Build history of the part. All positions in model axes, mm. A direction names the side the tool comes from. Round coordinates to 2 decimals unless told otherwise and drop trailing zeros. Loops run counter-clockwise (first coordinate to the right, second up) from the corner with the lowest first, then second, coordinate; pieces in that order, holes last. Notation, with made-up numbers: (54, 55.25) -> (63, 55.25) arc R25 cw to (63, 74.25) -> close; hole circle Ø11 at (12.5, 43). An arc over 180 degrees is marked (long way). Put each result on its own line as item: value. Start each with the question number.
Item 1: Cut at D-D, the plane y = -7. List the corners of the cut face in (x, z), plus the area to 3 significant figures.
Item 2: Drill centre lines: probe 1 along X at (y, z) = (-6, -3.5); probe 2 along X at (y, z) = (-11.5, -10.5); probe 3 along Y at (x, z) = (13, 7). Where is each one in solid material? Low to high. Write a range as [from, to].
Item 3: Cut at B-B, the plane z = -8. List the corners of the cut face in (x, y).
Item 4: Flat gauge pins, fed straight in: pin 1 Ø10 at (x, z) = (32, -7) entering from +Y; pin 2 Ø8 at (x, z) = (14, 4) entering from +Y; pin 3 Ø6 at (x, y) = (22.5, 5) entering from +Z. Where does each tip first touch, or does it go through?
Item 5: Cut at C-C, the plane x = -14.5. List the corners of the cut face in (y, z).
Item 6: Tool access for faces 1 (the cylindrical face through (-19.712, 0.165, -3.746)), 2 (the flat face through (40, -9.4, 0)), 3 (the flat face through (30, -8, 3)): list every direction of +Z, -Z, +X, -X, +Y, -Y with a clear straight run to the whole face (end or side of a thin tool).
Item 7: Cut at A-A, the plane y = 0. List the corners of the cut face in (x, z).
```python
from build123d import *

# Parameters (mm, degrees)
SKETCH1_R           = 18.5
BOSS_EXTRUDE1_DEPTH = 24
SKETCH2_R           = 16
BOSS_EXTRUDE2_DEPTH = 17
SKETCH4_R           = 6
BOSS_EXTRUDE3_DEPTH = 6
SKETCH5_R           = 3
BOSS_EXTRUDE4_DEPTH = 15
SKETCH6_W           = 6.457083565
SKETCH6_H           = 2.403469994
CUT_EXTRUDE1_DEPTH  = 11
SKETCH7_R           = 3.75
BOSS_EXTRUDE5_DEPTH = 5.5


with BuildPart() as part:
    # Sketch1 → Boss-Extrude1 (new body)
    with BuildSketch(Plane(origin=(0, 0, 0), x_dir=(0, 0, -1), z_dir=(1, 0, 0))):
        Circle(SKETCH1_R)
    extrude(amount=BOSS_EXTRUDE1_DEPTH)

    # Sketch2 → Boss-Extrude2 (add)
    with BuildSketch(Plane.ZY):
        Circle(SKETCH2_R)
    extrude(amount=BOSS_EXTRUDE2_DEPTH)

    # Sketch4 → Boss-Extrude3 (add)
    with BuildSketch(Plane(origin=(24, 0, 0), x_dir=(0, 0, -1), z_dir=(1, 0, 0))):
        with Locations((0, -7)):
            Circle(SKETCH4_R)
    extrude(amount=BOSS_EXTRUDE3_DEPTH)

    # Sketch5 → Boss-Extrude4 (add)
    with BuildSketch(Plane(origin=(30, 0, 0), x_dir=(0, 0, -1), z_dir=(1, 0, 0))):
        with Locations((0, -7)):
            Circle(SKETCH5_R)
    extrude(amount=BOSS_EXTRUDE4_DEPTH)

    # Sketch6 → Cut-Extrude1 (cut)
    with BuildSketch(Plane(origin=(45, 0, 0), x_dir=(0, 0, -1), z_dir=(1, 0, 0))):
        with Locations((-0.362875994, -10.601734997)):
            Rectangle(SKETCH6_W, SKETCH6_H)
    extrude(amount=-CUT_EXTRUDE1_DEPTH, mode=Mode.SUBTRACT)

    # Sketch7 → Boss-Extrude5 (add)
    with BuildSketch(Plane.ZY.offset(17)):
        Circle(SKETCH7_R)
    extrude(amount=BOSS_EXTRUDE5_DEPTH)


solid = part.part
```
Reply:
1. outline: (-17, -14.39) -> (0, -14.39) -> (0, -17.12) -> (24, -17.12) -> (24, -6) -> (30, -6) -> (30, -3) -> (45, -3) -> (45, 3) -> (30, 3) -> (30, 6) -> (24, 6) -> (24, 17.12) -> (0, 17.12) -> (0, 14.39) -> (-17, 14.39) -> close
1. area: 1,470 mm^2
2. probe 1: x = [-17, 30]
2. probe 2: x = [-17, 24]
2. probe 3: y = [-17.12, 17.12]
3. outline: (-17, -13.86) -> (0, -13.86) -> (0, -16.68) -> (24, -16.68) -> (24, 16.68) -> (0, 16.68) -> (0, 13.86) -> (-17, 13.86) -> close
4. pin 1: stops at y = -1.51
4. pin 2: stops at y = 18.5
4. pin 3: stops at z = 18.39
5. outline: circle Ø32 at (0, 0)
6. face 1: -X
6. face 2: +Z, -Z, +X, -Y
6. face 3: +X
7. outline: (-22.5, -3.75) -> (-17, -3.75) -> (-17, -16) -> (0, -16) -> (0, -18.5) -> (24, -18.5) -> (24, 18.5) -> (0, 18.5) -> (0, 16) -> (-17, 16) -> (-17, 3.75) -> (-22.5, 3.75) -> close
